```python
from build123d import *

# Parameters (mm, degrees)
F0_W      = 85
F0_H      = 19.05
F1_DEPTH  = 6.35
F2_R      = 1.6
F3_DEPTH  = 5
F4_R      = 2.5
F5_R      = 3
F6_R      = 3
F7_R      = 3
F8_R      = 4.75
F9_DEPTH  = 25
F10_R     = 1.6
F11_DEPTH = 25


with BuildPart() as f1:
    # F0 (on Front) → F1 (new body)
    with BuildSketch(Plane.XZ):
        Rectangle(F0_W, F0_H)
    extrude(amount=F1_DEPTH)

    # F2 (on face) → F3 (cut)
    with BuildSketch(Plane(origin=(0, 0, -9.525), x_dir=(1, 0, 0), z_dir=(0, 0, -1))):
        with Locations((25.5, 3.175)):
            Circle(F2_R)
        with Locations((-25.5, 3.175)):
            Circle(F2_R)
    extrude(amount=-F3_DEPTH, mode=Mode.SUBTRACT)

    # F4
    f4_edges = [f1.edges().sort_by_distance(p)[0] for p in [
        (-42.5, -3.175, 9.525),
    ]]
    fillet(f4_edges, radius=F4_R)

    # F5
    f5_edges = [f1.edges().sort_by_distance(p)[0] for p in [
        (42.5, -3.175, 9.525),
    ]]
    fillet(f5_edges, radius=F5_R)

    # F6
    f6_edges = [f1.edges().sort_by_distance(p)[0] for p in [
        (42.5, -3.175, -9.525),
    ]]
    fillet(f6_edges, radius=F6_R)

    # F7
    f7_edges = [f1.edges().sort_by_distance(p)[0] for p in [
        (-42.5, -3.175, -9.525),
    ]]
    fillet(f7_edges, radius=F7_R)

    # F8 (on face) → F9 (cut)
    with BuildSketch(Plane.XZ.offset(6.35)):
        with Locations((32.5, 0)):
            Circle(F8_R)
    extrude(amount=-F9_DEPTH, mode=Mode.SUBTRACT)

    # F10 (on face) → F11 (cut)
    with BuildSketch(Plane.XZ.offset(6.35)):
        with Locations((-15.501157, 0)):
            Circle(F10_R)
    extrude(amount=-F11_DEPTH, mode=Mode.SUBTRACT)


solid = f1.part
```
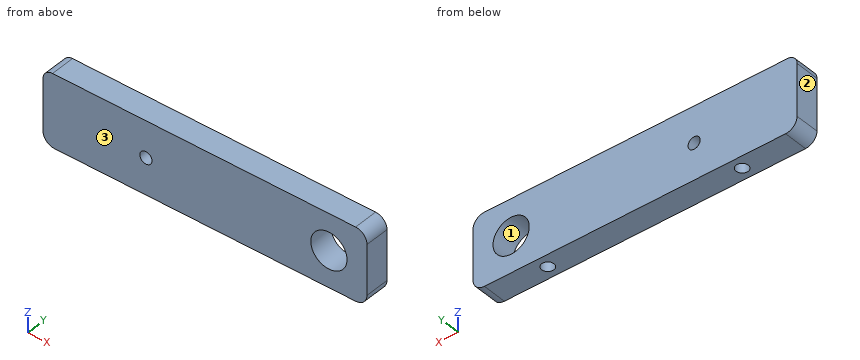
The listing builds one solid part. Answer for the finished solid, in the listing's coordinates (mm). Face numbers are marked on the shaded views. Coordinates: 2 decimals unless noted, no trailing zeros. Write each loop counter-clockwise with the first axis right and the second up, starting at its lowest first coordinate (ties: lowest second). Pieces come first, ordered by that corner, then holes. Notation, with made-up numbers: M -5,79.5 L 35,79.5 A36 ccw 35,118.5 Z; hole C -19,41.25 d2. An arc over 180 degrees is marked long. Use a Markdown table: item, result. Add a question column.
1. Section D-D (x = -25.5) is taken. Give the vertices of the cut face in (y, z) (3 decimals).
2. Given P1, Ø1, axis at x = -26, y = -2.5, coming from the -Z side (3 decimals); P2, Ø3, axis at x = -15.5, z = 0, coming from the +Y side, each flat-ended and moving along its own axis, determine where each tip first touches the part or whether it passes through.
3. Section A-A (z = 0) is taken. Give the vertices of the cut face in (x, y).
4. Section B-B (x = 32.5) is taken. Give the vertices of the cut face in (y, z) (3 decimals), plus the area to 3 significant figures.
5. Section C-C (y = -5.5) is taken. Give the vertices of the cut face in (x, z) (3 decimals).
6. For a pull along X with two mould halves and no side action, classify the marked faces 1, 2 and 3 as +X half, -X half, draft (parallel to the pull), parting line (faces both ways), or undercut.
7. Straight lines are drawn through the part: line 1 along Y through (x, z) = (25.5, -6.3) (3 decimals); line 2 along X through (y, z) = (-0.5, -0.25); line 3 along Z through (x, y) = (32.5, -3.25) (3 decimals). For each, find the intervals that lie inside material, in ascending order. Write a range as [from, to].
Data:
| question | item | result |
|---|---|---|
| 1 | outline | M -6.35,-9.525 L -4.775,-9.525 L -4.775,-4.525 L -1.575,-4.525 L -1.575,-9.525 L 0,-9.525 L 0,9.525 L -6.35,9.525 Z |
| 2 | P1 | stops at z = -4.525 |
| 2 | P2 | passes through |
| 3 | outline | M -42.5,-6.35 L -17.1,-6.35 L -17.1,0 L -42.5,0 Z; M -13.9,-6.35 L 27.75,-6.35 L 27.75,0 L -13.9,0 Z; M 37.25,-6.35 L 42.5,-6.35 L 42.5,0 L 37.25,0 Z |
| 4 | outline | M -6.35,-9.525 L 0,-9.525 L 0,-4.75 L -6.35,-4.75 Z; M -6.35,4.75 L 0,4.75 L 0,9.525 L -6.35,9.525 Z |
| 4 | area | 60.6 mm2 |
| 5 | outline | M -42.5,-6.525 A3 ccw -39.5,-9.525 L 39.5,-9.525 A3 ccw 42.5,-6.525 L 42.5,6.525 A3 ccw 39.5,9.525 L -40,9.525 A2.5 ccw -42.5,7.025 Z; hole C -15.501,0 d3.2; hole C 32.5,0 d9.5 |
| 6 | face 1 | undercut |
| 6 | face 2 | -X half |
| 6 | face 3 | draft |
| 7 | line 1 | y = [-6.35, -4.775], [-1.575, 0] |
| 7 | line 2 | x = [-42.5, -17.08], [-13.92, 27.76], [37.24, 42.5] |
| 7 | line 3 | z = [-9.525, -4.75], [4.75, 9.525] |
